from build123d import *

# Parameters (mm, degrees)
EXTRUDE_BASE_DEPTH              = 35
SKETCH2_R                       = 2.2
SKETCH2_R_2                     = 2.2479
CUT_BOLT_HOLES_DEPTH            = 10
CUT_BOLT_HEAD_INSETS_DEPTH      = 13
CUT_BOLT_HEAD_INSETS_DEPTH_BACK = 4.2
SKETCH3_R                       = 4.215
SKETCH4_W                       = 40
SKETCH4_H                       = 3
CUT_TOP_CLEARANCE_SLOT_DEPTH    = 45
FILLET_CLEARANCE_SLOT_PT_1_R    = 3
FILLET_CLEARANCE_SLOT_PT_2_R    = 3
BOSS_EXTRUDE1_DEPTH             = 6
BOSS_EXTRUDE2_START             = 6
BOSS_EXTRUDE2_DEPTH             = 6
SKETCH9_R                       = 2.2479
BOSS_EXTRUDE3_DEPTH             = 10
FILLET1_R                       = 0.5
CUT_EXTRUDE1_REACH              = 103.769
SKETCH10_W                      = 7
SKETCH10_H                      = 12.215570114
FILLET2_R                       = 0.5
CUT_EXTRUDE2_START              = -35
SKETCH11_W                      = 33.244666378
SKETCH11_H                      = 11
CUT_EXTRUDE2_DEPTH              = 35
SKETCH13_W                      = 28
SKETCH13_H                      = 10.000570114
CUT_EXTRUDE5_DEPTH              = 6
FILLET3_R                       = 5
SKETCH14_W                      = 3
SKETCH14_H                      = 12.5
BOSS_EXTRUDE4_DEPTH             = 3
SKETCH15_W                      = 9
SKETCH15_H                      = 1.5
CUT_EXTRUDE6_DEPTH              = 10
CUT_EXTRUDE7_DEPTH              = 6


# Some blends are built 0.0001 mm under size
with BuildPart() as part:
    # Sketch1 → Extrude-Base (new, symmetric)
    with BuildSketch(Plane.XY):
        Polygon((-14, 0), (0, 0), (0, -35), (-90, -35), (-90, -29), (-81, -29), (-81, -13), (-85, -13), (-85, -11), (-78, -11), (-78, -29), (-4, -29), (-4, -4), (-14, -4), align=None)
    extrude(amount=EXTRUDE_BASE_DEPTH, both=True)

    # Sketch2 → Cut-Bolt Holes (cut)
    with BuildSketch(Plane(origin=(0, -29, 0), x_dir=(1, 0, 0), z_dir=(0, 1, 0))):
        with Locations(Location((-12, -10, 0), (0, 0, 270))):
            Circle(SKETCH2_R)
        with Locations(Location((-12, 10, 0), (0, 0, 180))):
            Circle(SKETCH2_R)
        with Locations(Location((-40.244666378, 29.250570114, 0), (0, 0, 270))):
            Circle(SKETCH2_R_2)
        with Locations(Location((-40.244666378, -29.249429886, 0), (0, 0, 270))):
            Circle(SKETCH2_R_2)
        with Locations(Location((-85.244666378, 27.000570114, 0), (0, 0, 270))):
            Circle(SKETCH2_R)
        with Locations(Location((-85.244666378, -26.999429886, 0), (0, 0, 270))):
            Circle(SKETCH2_R)
    extrude(amount=-CUT_BOLT_HOLES_DEPTH, mode=Mode.SUBTRACT)

    # Sketch3 → Cut-Bolt Head Insets (cut, two sides: drawn at the far end of the back side and taken through both)
    with BuildSketch(Plane(origin=(0, -29, 0), x_dir=(1, 0, 0), z_dir=(0, 1, 0)).offset(-CUT_BOLT_HEAD_INSETS_DEPTH_BACK)):
        with Locations((-12, -10)):
            Circle(SKETCH3_R)
        with Locations((-40.244666378, -29.249429886)):
            Circle(SKETCH3_R)
        with Locations((-85.244666378, -26.999429886)):
            Circle(SKETCH3_R)
        with Locations((-85.244666378, 27.000570114)):
            Circle(SKETCH3_R)
        with Locations(Location((-12, 10, 0), (0, 0, 90))):
            Circle(SKETCH3_R)
        with Locations(Location((-40.244666378, 29.249429886, 0), (0, 0, 90))):
            Circle(SKETCH3_R)
    extrude(amount=CUT_BOLT_HEAD_INSETS_DEPTH + CUT_BOLT_HEAD_INSETS_DEPTH_BACK, mode=Mode.SUBTRACT)

    # Sketch4 → Cut-Top Clearance Slot (cut)
    with BuildSketch(Plane.ZY.offset(90)):
        with Locations((0, -33.5)):
            Rectangle(SKETCH4_W, SKETCH4_H)
    extrude(amount=-CUT_TOP_CLEARANCE_SLOT_DEPTH, mode=Mode.SUBTRACT)

    # Fillet-Clearance Slot Pt 1
    fillet_clearance_slot_pt_1_edges = [part.edges().sort_by_distance(p)[0] for p in [
        (-67.5, -32, 20),
        (-67.5, -32, -20),
    ]]
    fillet(fillet_clearance_slot_pt_1_edges, radius=FILLET_CLEARANCE_SLOT_PT_1_R - 0.0001)  # a hair under: the kernel refuses the full size

    # Fillet-Clearance Slot Pt 2
    # the kernel refuses this fillet: 3 mm, written as the material it takes off along each edge
    with BuildSketch(Plane(origin=(-95.490486718, -35, 20), x_dir=(0, 0, 1), z_dir=(1, 0, 0))) as fillet_clearance_slot_pt_2_piece_1:
        with BuildLine():
            CenterArc((2.196194687, -3), FILLET_CLEARANCE_SLOT_PT_2_R, 90, 60.000551337)
            Line((-0.401895958, -1.500025), (-0.661705022, -1.3500275))
            ThreePointArc((-0.661705022, -1.3500275), (-0.3, -0.0001), (-0.3, 0))
            Line((-0.3, 0), (0, 0.3))
            Line((0, 0.3), (2.196194687, 0.3))
            Line((2.196194687, 0.3), (2.196194687, 0))
        make_face()
    extrude(amount=50.490486718, mode=Mode.SUBTRACT)
    with BuildSketch(Plane(origin=(-95.490486718, -35, -20), x_dir=(0, 0.9659313848535164, 0.2587982993664522), z_dir=(1, 0, 0))) as fillet_clearance_slot_pt_2_piece_2:
        with BuildLine():
            CenterArc((2.329422704, -2.897768274), FILLET_CLEARANCE_SLOT_PT_2_R, 105.000679234, 60.000551337)
            Line((-0.56837145, -2.121373376), (-0.858150866, -2.043733886))
            Line((-0.858150866, -2.043733886), (-0.289779415, 0.07763949))
            Line((-0.289779415, 0.07763949), (0.07763949, 0.289779415))
            ThreePointArc((0.07763949, 0.289779415), (0.077736083, 0.289753536), (1.475282068, 0.289776827))
            Line((1.475282068, 0.289776827), (1.552931216, 0))
        make_face()
    extrude(amount=50.490486718, mode=Mode.SUBTRACT)

    # Sketch5 → Boss-Extrude1 (add)
    with BuildSketch(Plane.XY.offset(35)):
        with BuildLine():
            Line((-78, -35), (-90, -35))
            Line((-90, -35), (-90, -32))
            Line((-90, -32), (-78, -32))
            ThreePointArc((-78, -32), (-76.5, -33.5), (-78, -35))
        make_face()
    extrude(amount=BOSS_EXTRUDE1_DEPTH)

    # Sketch7 → Boss-Extrude2 (add)
    with BuildSketch(Plane(origin=(0, 0, -35), x_dir=(-1, 0, 0), z_dir=(0, 0, -1)).offset(BOSS_EXTRUDE2_START)):
        with BuildLine():
            Line((78, -32), (90, -32))
            Line((90, -32), (90, -35))
            Line((90, -35), (78, -35))
            ThreePointArc((78, -35), (76.5, -33.5), (78, -32))
        make_face()
    extrude(amount=-BOSS_EXTRUDE2_DEPTH)

    # Sketch9 → Boss-Extrude3 (add)
    with BuildSketch(Plane(origin=(0, 0, 0), x_dir=(0, 0, -1), z_dir=(1, 0, 0))):
        with BuildLine():
            Line((25.000570114, 0), (-24.999429886, 0))
            Line((-24.999429886, 0), (-24.999429886, 2.5))
            ThreePointArc((-24.999429886, 2.5), (-22.070497698, 9.571067812), (-14.999429886, 12.5))
            Line((-14.999429886, 12.5), (15.000570114, 12.5))
            ThreePointArc((15.000570114, 12.5), (22.071637926, 9.571067812), (25.000570114, 2.5))
            Line((25.000570114, 2.5), (25.000570114, 0))
        make_face()
        with Locations(Location((-17.999429886, 5.5, 0), (0, 0, 90))):
            Circle(SKETCH9_R, mode=Mode.SUBTRACT)
        with Locations(Location((18.000570114, 5.5, 0), (0, 0, 90))):
            Circle(SKETCH9_R, mode=Mode.SUBTRACT)
    extrude(amount=-BOSS_EXTRUDE3_DEPTH)

    # Fillet1
    # the kernel refuses this fillet: 0.5 mm, written as the material it adds along each edge
    with BuildSketch(Plane(origin=(-78, -33.5, 35), x_dir=(0, 1, 0), z_dir=(-1, 0, 0))) as fillet1_piece_1_section:
        with BuildLine():
            CenterArc((1.5 + FILLET1_R, -FILLET1_R), FILLET1_R, 90, 90)
            Line((1.5, -FILLET1_R), (1.5, 0))
            Line((1.5, 0), (1.5 + FILLET1_R, 0))
        make_face()
    fillet1_piece_1 = revolve(axis=Axis((-78, -33.5, 35), (0, 0, -1)), revolution_arc=227.8232683, mode=Mode.PRIVATE)
    fillet1_piece_1 = split(fillet1_piece_1, bisect_by=Plane(origin=(-77.658393022, -35, 35.082006822), z_dir=(0, 1, 0)), keep=Keep.TOP, mode=Mode.PRIVATE)
    add(fillet1_piece_1)
    with BuildSketch(Plane(origin=(-90, -32, 35), x_dir=(0, 1, 0), z_dir=(1, 0, 0))) as fillet1_piece_2:
        with BuildLine():
            CenterArc((FILLET1_R, FILLET1_R), FILLET1_R, 180, 90)
            Line((0, FILLET1_R), (0, 0))
            Line((0, 0), (FILLET1_R, 0))
        make_face()
    extrude(amount=12)
    with BuildSketch(Plane(origin=(-78, -33.5, -35), x_dir=(-0.741077326598375, -0.6714196869334451, 0), z_dir=(-0.6714196869334451, 0.741077326598375, 0))) as fillet1_piece_3_section:
        with BuildLine():
            CenterArc((1.5 + FILLET1_R, -FILLET1_R), FILLET1_R, 90, 90)
            Line((1.5, -FILLET1_R), (1.5, 0))
            Line((1.5, 0), (1.5 + FILLET1_R, 0))
        make_face()
    fillet1_piece_3 = revolve(axis=Axis((-78, -33.5, -35), (0, 0, 1)), revolution_arc=227.8232683, mode=Mode.PRIVATE)
    fillet1_piece_3 = split(fillet1_piece_3, bisect_by=Plane(origin=(-76.494034021, -35, -35.2500003), z_dir=(0, 1, 0)), keep=Keep.TOP, mode=Mode.PRIVATE)
    add(fillet1_piece_3)
    with BuildSketch(Plane(origin=(-78, -32, -35), x_dir=(0, 0, -1), z_dir=(-1, 0, 0))) as fillet1_piece_4:
        with BuildLine():
            CenterArc((FILLET1_R, -FILLET1_R), FILLET1_R, 90, 90)
            Line((0, -FILLET1_R), (0, 0))
            Line((0, 0), (FILLET1_R, 0))
        make_face()
    extrude(amount=12)

    # Cut-Extrude1: up to this face of the body (flat: up to its plane)
    cut_extrude1_end = Plane(part.part.faces().sort_by_distance((-85.554984705, -29, 0.000122771))[0])
    # Sketch10 → Cut-Extrude1 (cut, up to the picked face)
    with BuildSketch(Plane(origin=(0, -11, 0), x_dir=(1, 0, 0), z_dir=(0, 1, 0)), mode=Mode.PRIVATE) as cut_extrude1_sk1:
        with Locations((-81.5, -28.892214943)):
            Rectangle(SKETCH10_W, SKETCH10_H)
    cut_extrude1_tool1 = split(extrude(cut_extrude1_sk1.sketch, amount=-CUT_EXTRUDE1_REACH, mode=Mode.PRIVATE), bisect_by=cut_extrude1_end, keep=Keep.BOTH, mode=Mode.PRIVATE)
    # Sketch10 → Cut-Extrude1 (cut, up to the picked face)
    with BuildSketch(Plane(origin=(0, -11, 0), x_dir=(1, 0, 0), z_dir=(0, 1, 0)), mode=Mode.PRIVATE) as cut_extrude1_sk2:
        Polygon((-85, 22.785570416), (-78, 22.784429886), (-78, 35), (-85, 35), align=None)
    cut_extrude1_tool2 = split(extrude(cut_extrude1_sk2.sketch, amount=-CUT_EXTRUDE1_REACH, mode=Mode.PRIVATE), bisect_by=cut_extrude1_end, keep=Keep.BOTH, mode=Mode.PRIVATE)
    add(cut_extrude1_tool1.solids().sort_by(Axis((-81.5, -11, 28.892215), (0, -1, 0)))[0], mode=Mode.SUBTRACT)
    add(cut_extrude1_tool2.solids().sort_by(Axis((-81.499946, -11, -28.8925), (0, -1, 0)))[0], mode=Mode.SUBTRACT)

    # Fillet2
    fillet2_edges = [part.edges().sort_by_distance(p)[0] for p in [
        (-78, -29, 0),
        (-79.5, -29, 22.784429886),
        (-79.5, -29, -22.784674285),
    ]]
    fillet(fillet2_edges, radius=FILLET2_R)

    # Sketch11 → Cut-Extrude2 (cut)
    with BuildSketch(Plane(origin=(0, 0, 0), x_dir=(1, 0, 0), z_dir=(0, 1, 0)).offset(CUT_EXTRUDE2_START)):
        with Locations((-16.622333189, -30.499429886)):
            Rectangle(SKETCH11_W, SKETCH11_H)
        with Locations((-16.622333189, 30.499429886)):
            Rectangle(SKETCH11_W, SKETCH11_H)
    extrude(amount=CUT_EXTRUDE2_DEPTH, mode=Mode.SUBTRACT)

    # Sketch13 → Cut-Extrude5 (cut)
    with BuildSketch(Plane(origin=(0, -29, 0), x_dir=(1, 0, 0), z_dir=(0, 1, 0))):
        with Locations((-61.244666378, -29.999714943)):
            Rectangle(SKETCH13_W, SKETCH13_H)
        with Locations((-61.244666378, 29.999714943)):
            Rectangle(SKETCH13_W, SKETCH13_H)
    extrude(amount=-CUT_EXTRUDE5_DEPTH, mode=Mode.SUBTRACT)

    # Fillet3
    fillet3_edges = [part.edges().sort_by_distance(p)[0] for p in [
        (-75.244666378, -32, 24.999429886),
        (-47.244666378, -32, 24.999429886),
        (-75.244666378, -32, -24.999429886),
        (-47.244666378, -32, -24.999429886),
    ]]
    fillet(fillet3_edges, radius=FILLET3_R)

    # Sketch14 → Boss-Extrude4 (add)
    with BuildSketch(Plane.ZY.offset(10)):
        with Locations((12.033169886, 6.25)):
            Rectangle(SKETCH14_W, SKETCH14_H)
        with Locations((-12.033169886, 6.25)):
            Rectangle(SKETCH14_W, SKETCH14_H)
    extrude(amount=BOSS_EXTRUDE4_DEPTH)

    # Sketch15 → Cut-Extrude6 (cut)
    with BuildSketch(Plane(origin=(0, -32, 0), x_dir=(1, 0, 0), z_dir=(0, 1, 0))):
        with Locations((-81, -38.25)):
            Rectangle(SKETCH15_W, SKETCH15_H)
    cut_extrude6 = extrude(amount=-CUT_EXTRUDE6_DEPTH, mode=Mode.SUBTRACT)

    # Mirror1: Cut-Extrude6 across plane
    add(cut_extrude6.mirror(Plane.XY), mode=Mode.SUBTRACT)

    # Sketch16 → Cut-Extrude7 (cut)
    with BuildSketch(Plane.ZY.offset(10)):
        Polygon((-18.000570114, 0.4), (-13.583840555, 2.95), (-13.583840555, 8.05), (-18.000570114, 10.6), (-22.417299673, 8.05), (-22.417299673, 2.95), align=None)
        Polygon((22.417299673, 2.95), (18.000570114, 0.4), (13.583840555, 2.95), (13.583840555, 8.05), (18.000570114, 10.6), (22.417299673, 8.05), align=None)
    extrude(amount=-CUT_EXTRUDE7_DEPTH, mode=Mode.SUBTRACT)


solid = part.part
Verification items for the finished model (mm, model axes). A direction names the side the tool comes from. Coordinates: 2 decimals unless noted, no trailing zeros. Order: outer loops, then holes, each group sorted by start corner. A loop starts at its lowest first (then second) coordinate and runs counter-clockwise, first axis right, second up. Notation, with made-up numbers: M 61.25,79 L 85.25,79 A36 ccw 85.25,116 Z; hole C -14,81.5 d8. An arc over 180 degrees is marked long. One line per item, written item: value. Start each with the question number.
Item 1: Scan lines: probe 1 along X at (y, z) = (-27.5, 10); probe 2 along X at (y, z) = (-34, 10); probe 3 along Z at (x, y) = (-6, 7.5). Record each from-to range of solid material in increasing order.
Item 2: Access from +Z, -Z, +X, -X, +Y, -Y to the whole of each face (thin tool, end or side, straight path). Record for faces 1 (the flat face through (-7.042, 1.693, 20.24)), 2 (the flat face through (-68, -32, 0)), 3 (the flat face through (-75.245, -32, 33)), 4 (the flat face through (-84, -32, 37)).
Item 3: Sectioned sample at A-A (y = -26). Enter the section's corners in (x, z).
Item 4: Mould release check, pull along X, two halves, no side actions. Record for faces 5 (the flat face through (-85, -12, 0)), 6 (the flat face through (-7, 5, 13.584)), 7 (the flat face through (-47.245, -32, 33)): released by +X, released by -X, zero draft, split by the parting line, or undercut.
Item 5: Gauge pin test, flat ends, axial feed: pin 1 (0.6 mm diameter, centred on y = -12, z = -7, fed in from -X); pin 2 (5.5 mm diameter, centred on y = 8.5, z = 19, fed in from -X); pin 3 (6.5 mm diameter, centred on x = -85.24, z = 27, fed in from +Y); pin 4 (8 mm diameter, centred on y = -6, z = -32.5, fed in from -X). Record the tip position at first contact, or that the pin passes through.
Item 6: Sectioned sample at B-B (y = 5.5). Enter the section's corners in (x, z).
Item 7: Sectioned sample at C-C (x = -29.5). Enter the section's corners in (y, z).
Conclusion:
1. probe 1: x = -81 to -78, -4 to 0
1. probe 2: x = -45 to -14.2, -9.8 to 0
1. probe 3: z = -23.66 to -22.42, -13.58 to 13.58, 22.42 to 23.66
2. face 1: -X
2. face 2: -X, -Y
2. face 3: +Z, +Y, -Y
2. face 4: +Z, +X, -X, +Y
3. outline: M -81,-22.78 L -78,-22.78 L -78,22.78 L -81,22.78 Z; M -4,-25 L 0,-25 L 0,25 L -4,25 Z
4. face 5: released by -X
4. face 6: zero draft
4. face 7: undercut
5. pin 1: stops at x = -85
5. pin 2: stops at x = -10
5. pin 3: stops at y = -33.2
5. pin 4: passes through
6. outline: M -13,-13.53 L -10,-13.53 L -10,-13.58 L -4,-13.58 L -4,-15.75 L 0,-15.75 L 0,15.75 L -4,15.75 L -4,13.58 L -10,13.58 L -10,13.53 L -13,13.53 L -13,10.53 L -10,10.53 L -10,-10.53 L -13,-10.53 Z; M -10,-24.54 L 0,-24.54 L 0,-20.25 L -4,-20.25 L -4,-22.42 L -10,-22.42 Z; M -10,22.42 L -4,22.42 L -4,20.25 L 0,20.25 L 0,24.54 L -10,24.54 Z
7. outline: M -35,-25 L -29,-25 L -29,25 L -35,25 Z
